Here's how the part is built. I have some questions about the finished solid (model axes, mm). A direction names the side the tool comes from. Round coordinates to 2 decimals unless told otherwise and drop trailing zeros. Loops run counter-clockwise (first coordinate to the right, second up) from the corner with the lowest first, then second, coordinate; pieces in that order, holes last. Notation, with made-up numbers: (64, -1) - (101, -1) arc R13 ccw to (101, 21) - close; hole circle Ø2 at (79, 80). An arc over 180 degrees is marked (long way). Answer as a JSON object with one key per item and string values. Group by question number.
1) I want a section at A-A, the plane x = -4. Please give me the cut outline in (y, z).
2) I want a section at B-B, the plane z = 2. Please give me the cut outline in (x, y).
3) I want a section at C-C, the plane z = 5.3. Please give me the cut outline in (x, y).
4) If I drill on line 1 along Y through (x, z) = (-8.5, 1.45); line 2 along Z through (x, y) = (-10.75, -4.5); line 3 along X through (y, z) = (-4, 1.3), over which ranges is the centre line in solid material (lowest first)? Write a range as [from, to].
5) If we mould it in two halves opening along X, with no side actions, what happens to faces 3 (the face through (-4, -9.543, 2)), 4 (the face through (-3.683, -3.01, 2.095)), 5 (the face through (-0.74, -1.38, 2.85))? For each: pulls with the +X half, pulls with the -X half, needs draft (parallel to the pull), parting line crosses it, or undercut.
6) Will these pins go through, and if not, where does the flat tip stop? P1, Ø1, axis at y = 2, z = 2.5, coming from the -X side; P2, Ø1.5, axis at x = -12, y = -3.5, coming from the -Z side; P3, Ø1, axis at x = -14, z = 4, coming from the -Y side.
7) Which directions (+Z, -Z, +X, -X, +Y, -Y) give clear straight access to the entire face, cutting with the end or side of a thin tool? Please do faces 1 (the face through (-9, -1, 4.25)), 2 (the face through (-4, 6.557, 2)).
Autodesk Inventor part; units mm, degrees
ref_plane "YZ Plane" through (0, 0, 0) normal (1, 0, 0) x (0, 1, 0)
ref_plane "XZ Plane" through (0, 0, 0) normal (0, 1, 0) x (-1, 0, 0)
ref_plane "XY Plane" through (0, 0, 0) normal (0, 0, 1) x (1, 0, 0)
sketch "Szkic1" plane through (0, 0, 0) normal (0, 0, 1) x (1, 0, 0)
  line L0 (0, 6.5573) -> (0, -9.5427)
  circle A0 centre (-8.5, -1.4927) radius 5.05
  arc A1 (-8.5, 6.5573) -> (-8.5, -9.5427) centre (-8.5, -1.4927) ccw
  line L1 (0, 6.5573) -> (-8.5, 6.5573)
  line L2 (0, -9.5427) -> (-8.5, -9.5427)
  point P0 (0, 0)
  dimension "d0" = 16.1
  dimension "d1" = 8.5
  dimension "d2" = 10.1
  dimension "d3" = 8.05
  dimension "d4" = 3
extrude "Wyciągnięcie proste1" add sketch "Szkic1" along normal blind 6 contours L0 L2 A1 L1 | A0
chamfer "Faza1" distance 2 distance2 5 1 edges at (0, -1.4927, 6) measured on face at (-2.8333, -4.176, 6)
extrude "Wyciągnięcie proste2" cut sketch "Szkic1" along normal blind 4.25 contours A0
fillet "Zaokrąglenie1" radius 2 4 edges at (-16.55, -1.4927, 6) (-5.25, -9.5427, 6) (-5.25, 6.5573, 6) (-2, -1.4927, 6)
equation "\"d3\" = 0.5 * d0"
properties part number "3DP_ABS_Front_Door_Magnet_Holder"
Outcome:
{
 "1": {"outline": "(-9.54, 0) - (-3.78, 0) - (-3.78, 4.25) - (0.8, 4.25) - (0.8, 0) - (6.56, 0) - (6.56, 4) arc R2 ccw to (4.56, 6) - (-7.54, 6) arc R2 ccw to (-9.54, 4) - close"},
 "2": {"outline": "(-8.5, -9.54) - (-0.4, -9.54) - (-0.4, 6.56) - (-8.5, 6.56) arc R8.05 ccw to start; hole circle Ø10.1 at (-8.5, -1.49)"},
 "3": {"outline": "(-8.5, -9.06) - (-1.83, -9.06) - (-1.83, 6.08) - (-8.5, 6.08) arc R7.57 ccw to start"},
 "4": {"line 1": "[-9.54, -6.54], [3.56, 6.56]", "line 2": "[4.25, 6]", "line 3": "[-16.15, -12.88], [-4.12, -0.12]"},
 "5": {"face 3": "needs draft", "face 4": "undercut", "face 5": "pulls with the +X half"},
 "6": {"P1": "x = -15.97", "P2": "z = 4.25", "P3": "y = -7.8"},
 "7": {"face 1": "-Z", "face 2": "+Z, -Z, +X, -X, +Y"}
}
